Geometry check sheet. Reference: the model listing, model coordinates, mm. Give positions to 0.01 mm unless a question says otherwise; leave off trailing zeros. Loops run counter-clockwise (first coordinate to the right, second up) from the corner with the lowest first, then second, coordinate; pieces in that order, holes last. Notation, with made-up numbers: (-40, 40) - (-18, 40) arc R24 cw to (-18, 60) - close; hole circle Ø3 at (87, -3.5). An arc over 180 degrees is marked (long way). Use a Markdown table: item, result. Add a question column.
1. Depth check by flat-ended pin: P1, Ø5, axis at x = 19.5, y = -136, coming from the -Z side; P2, Ø1, axis at y = -412, z = 56.5, coming from the +X side; P3, Ø5, axis at x = -3, y = -279, coming from the -Z side. Enter the tip coordinate at first touch or a pass-through.
2. Material ranges on L1, parallel to Z at x = 12, y = -265.5; L2, parallel to Z at x = -33, y = -108; L3, parallel to X at y = -280, z = 20, recorded low to high.
3. Cross-section at A-A on y = -159. Enter the section's corners in (x, z), and give its area (3 significant figures).
from build123d import *


with BuildPart() as part:
    # Sketch → AdditiveLoft section 0
    with BuildSketch(Plane.XZ):
        with BuildLine():
            ThreePointArc((-50, 100), (-36.803399, 44.098301), (0, 0))
            ThreePointArc((0, 0), (36.803399, 44.098301), (50, 100))
            Line((-50, 100), (50, 100))
        make_face()
    # Sketch003 (on DatumPlane) → AdditiveLoft section 1
    with BuildSketch(Plane.XZ.offset(200)):
        with BuildLine():
            Line((-50, 100), (50, 100))
            ThreePointArc((0, 0), (36.803399, 44.098301), (50, 100))
            ThreePointArc((-50, 100), (-36.803399, 44.098301), (0, 0))
        make_face()
    # Sketch001 (on DatumPlane) → AdditiveLoft section 2
    with BuildSketch(Plane.XZ.offset(350)):
        with BuildLine():
            Line((-34.658561, 100), (34.658561, 100))
            ThreePointArc((0, 20), (25.621549, 56.407524), (34.658561, 100))
            ThreePointArc((-34.658561, 100), (-25.621549, 56.407524), (0, 20))
        make_face()
    # Sketch002 (on DatumPlane) → AdditiveLoft section 3
    with BuildSketch(Plane.XZ.offset(500)):
        with BuildLine():
            Line((-2.620873, 100), (2.620873, 100))
            ThreePointArc((0, 80), (1.962866, 89.914503), (2.620873, 100))
            ThreePointArc((-2.620873, 100), (-1.962866, 89.914503), (0, 80))
        make_face()
    loft(ruled=True)


solid = part.part
Values found:
| question | item | result |
|---|---|---|
| 1 | P1 | stops at z = 15.38 |
| 1 | P2 | stops at x = 9.27 |
| 1 | P3 | stops at z = 10.93 |
| 2 | L1 | z = 20.02 to 100 |
| 2 | L2 | z = 37.06 to 100 |
| 2 | L3 | x = -9.95 to 9.95 |
| 3 | outline | (-50, 100) arc R125 ccw to (0, 0) arc R125 ccw to (50, 100) - close |
| 3 | area | 6,990 mm2 |
